Input: part model. Units: mm. Frame: model coordinates. A direction names the side the tool comes from. Give positions to 0.01 mm unless a question says otherwise; leave off trailing zeros. Write each loop counter-clockwise with the first axis right and the second up, starting at its lowest first coordinate (ties: lowest second). Pieces come first, ordered by that corner, then holes. Notation, with made-up numbers: (13, -3.75) -> (46, -3.75) arc R16 cw to (46, 24.25) -> close; hole circle Ø5 at (-6, 63.25). An arc over 180 degrees is marked (long way). Return JSON: item names as keys, results as strings. Group by question number.
Item 1: Section B-B, the plane z = -15. Return loops of the section in (x, y).
Item 2: Section D-D, the plane y = 1.4. Count the separate pieces of the cut face and the enclosed holes in it, then the cut area to 3 significant figures.
Item 3: Section A-A, the plane z = 9. Return loops of the section in (x, y).
Item 4: Line query: line 1 (X direction, y = 1.3, z = -8); line 2 (X direction, y = 0.4, z = 33); line 3 (Z direction, x = 49.5, y = 1.6). Output: solid intervals per line, ascending. Write a range as [from, to].
Item 5: Pin query (flat end, axial travel): P1, Ø2, axis at x = -27.5, y = 2, coming from the -Z side; P2, Ø1.5, axis at y = 1.5, z = -10, coming from the -X side; P3, Ø1.5, axis at x = -35, y = 2, coming from the +Z side. Return the tip coordinate at first contact, or that it passes through.
Item 6: Section C-C, the plane x = -36. Return loops of the section in (y, z), then the cut area to 3 significant figures.
Item 7: Set-up query: faces 3 (the face through (-29, 2, 19.827)), 4 (the face through (49, 2, -17.473)). Return all of +Z, -Z, +X, -X, +Y, -Y with unobstructed straight access to the full face (end or side cutting, diameter ignored); none if empty.
Item 8: Mould query, pull axis Z, two halves, no side actions, for faces 1 (the face through (73, 2, 41.827)), 2 (the face through (85.873, 2, -12)). Classes: released by +Z, released by -Z, zero draft, split by the parting line, or undercut.
from build123d import *

# Parameters (mm, degrees)
SKETCH_1_R      = 5.1
SKETCH_1_R_2    = 7.5
SKETCH_1_W      = 5
SKETCH_1_H      = 10
EXTRUDE_1_DEPTH = 5


with BuildPart() as part:
    # 草图1 → 凸台-拉伸1 (new body)
    with BuildSketch(Plane(origin=(0, 0, 0), x_dir=(1, 0, 0), z_dir=(0, 1, 0))):
        with BuildLine():
            Line((41.226602941, -22.421259901), (43.51896829, -39.231939129))
            ThreePointArc((43.51896829, -39.231939129), (44.518645935, -41.086690093), (46.491458794, -41.826599515))
            Line((46.491458794, -41.826599515), (46.872785616, -41.826599515))
            Line((46.872785616, -41.826599515), (100.872785616, -41.826599515))
            Line((100.872785616, -41.826599515), (100.872785616, -21.15))
            Line((100.872785616, -21.15), (100.872785616, 22.473400485))
            Line((100.872785616, 22.473400485), (46.393557665, 22.473400485))
            ThreePointArc((46.393557665, 22.473400485), (44.463634871, 21.770223946), (43.438429698, 19.990332491))
            Line((43.438429698, 19.990332491), (41.307141533, 7.806468479))
            ThreePointArc((41.307141533, 7.806468479), (40.28193636, 6.026577025), (38.352013566, 5.323400485))
            Line((38.352013566, 5.323400485), (-80.606442335, 5.323400485))
            ThreePointArc((-80.606442335, 5.323400485), (-82.536365129, 6.026577025), (-83.561570302, 7.806468479))
            Line((-83.561570302, 7.806468479), (-85.692858467, 19.990332491))
            ThreePointArc((-85.692858467, 19.990332491), (-86.71806364, 21.770223946), (-88.647986434, 22.473400485))
            Line((-88.647986434, 22.473400485), (-94.127214384, 22.473400485))
            Line((-94.127214384, 22.473400485), (-94.127214384, 17.473400485))
            Line((-94.127214384, 17.473400485), (-89.127214384, 17.473400485))
            Line((-89.127214384, 17.473400485), (-89.127214384, 7.473400485))
            Line((-89.127214384, 7.473400485), (-94.127214384, 7.473400485))
            Line((-94.127214384, 7.473400485), (-94.127214384, -4.826599515))
            Line((-94.127214384, -4.826599515), (-89.127214384, -4.826599515))
            Line((-89.127214384, -4.826599515), (-89.127214384, -14.826599515))
            Line((-89.127214384, -14.826599515), (-94.127214384, -14.826599515))
            Line((-94.127214384, -14.826599515), (-94.127214384, -19.826599515))
            Line((-94.127214384, -19.826599515), (38.254112437, -19.826599515))
            ThreePointArc((38.254112437, -19.826599515), (40.226925296, -20.566508937), (41.226602941, -22.421259901))
        make_face()
        with Locations(Location((57.372785616, -30.826599515, 0), (0, 0, 270))):
            Circle(SKETCH_1_R, mode=Mode.SUBTRACT)
        with Locations(Location((89.372785616, -30.826599515, 0), (0, 0, 270))):
            Circle(SKETCH_1_R_2, mode=Mode.SUBTRACT)
        with Locations((49.372785616, 12.473400485)):
            Rectangle(SKETCH_1_W, SKETCH_1_H, mode=Mode.SUBTRACT)
        with Locations((49.372785616, -9.826599515)):
            Rectangle(SKETCH_1_W, SKETCH_1_H, mode=Mode.SUBTRACT)
        with Locations((83.372785616, -9.826599515)):
            Rectangle(SKETCH_1_W, SKETCH_1_H, mode=Mode.SUBTRACT)
        with Locations((83.372785616, 12.473400485)):
            Rectangle(SKETCH_1_W, SKETCH_1_H, mode=Mode.SUBTRACT)
        with BuildLine():
            ThreePointArc((52.497785616, -22.382851828), (50.478494499, -23.932308398), (48.929037929, -25.951599515))
            ThreePointArc((48.929037929, -25.951599515), (49.569582385, -28.342143972), (51.960126842, -27.701599515))
            ThreePointArc((51.960126842, -27.701599515), (52.953368233, -26.407182132), (54.247785616, -25.413940741))
            ThreePointArc((54.247785616, -25.413940741), (54.888330072, -23.023396285), (52.497785616, -22.382851828))
        make_face(mode=Mode.SUBTRACT)
        with BuildLine():
            ThreePointArc((65.816533303, -25.951599503), (64.267076731, -23.932308389), (62.247785614, -22.38285182))
            ThreePointArc((62.247785614, -22.38285182), (59.857241158, -23.023396278), (60.497785616, -25.413940734))
            ThreePointArc((60.497785616, -25.413940734), (61.792202999, -26.407182125), (62.785444391, -27.701599506))
            ThreePointArc((62.785444391, -27.701599506), (65.175988849, -28.34214396), (65.816533303, -25.951599503))
        make_face(mode=Mode.SUBTRACT)
        with BuildLine():
            ThreePointArc((62.247785626, -39.270347195), (64.267076742, -37.720890621), (65.81653331, -35.701599501))
            ThreePointArc((65.81653331, -35.701599501), (65.175988849, -33.311055045), (62.785444394, -33.951599506))
            ThreePointArc((62.785444394, -33.951599506), (61.792203004, -35.24601689), (60.497785622, -36.239258284))
            ThreePointArc((60.497785622, -36.239258284), (59.857241169, -38.629802741), (62.247785626, -39.270347195))
        make_face(mode=Mode.SUBTRACT)
        with BuildLine():
            ThreePointArc((48.929037937, -35.701599515), (50.478494509, -37.720890632), (52.497785627, -39.270347201))
            ThreePointArc((52.497785627, -39.270347201), (54.888330083, -38.629802742), (54.247785624, -36.239258286))
            ThreePointArc((54.247785624, -36.239258286), (52.953368241, -35.246016896), (51.960126849, -33.951599514))
            ThreePointArc((51.960126849, -33.951599514), (49.569582392, -33.311055058), (48.929037937, -35.701599515))
        make_face(mode=Mode.SUBTRACT)
    extrude(amount=EXTRUDE_1_DEPTH)


solid = part.part
Answer below:
{
 "1": {"outline": "(-89.13, 0) -> (-84.82, 0) -> (-84.82, 5) -> (-89.13, 5) -> close; (42.57, 0) -> (46.87, 0) -> (46.87, 5) -> (42.57, 5) -> close; (51.87, 0) -> (80.87, 0) -> (80.87, 5) -> (51.87, 5) -> close; (85.87, 0) -> (100.87, 0) -> (100.87, 5) -> (85.87, 5) -> close"},
 "2": {"separate pieces": "1", "enclosed holes": "10", "area": "6,700 mm2"},
 "3": {"outline": "(-89.13, 0) -> (46.87, 0) -> (46.87, 5) -> (-89.13, 5) -> close; (51.87, 0) -> (80.87, 0) -> (80.87, 5) -> (51.87, 5) -> close; (85.87, 0) -> (100.87, 0) -> (100.87, 5) -> (85.87, 5) -> close"},
 "4": {"line 1": "x = [-89.13, -83.6], [41.34, 46.87], [51.87, 80.87], [85.87, 100.87]", "line 2": "x = [42.67, 52.76], [61.99, 82.19], [96.55, 100.87]", "line 3": "z = [-22.47, -17.47], [-7.47, 4.83], [14.83, 25.07], [28.3, 33.35], [36.58, 41.83]"},
 "5": {"P1": "stops at z = -5.32", "P2": "stops at x = -89.13", "P3": "stops at z = 19.83"},
 "6": {"outline": "(0, -5.32) -> (5, -5.32) -> (5, 19.83) -> (0, 19.83) -> close", "area": "126 mm2"},
 "7": {"face 3": "+Z, -X, +Y, -Y", "face 4": "+Y, -Y"},
 "8": {"face 1": "released by +Z", "face 2": "undercut"}
}
